Read the model definition and answer for the solid it produces. Units are mm, in the model's axes. Give positions to 0.01 mm unless a question says otherwise; leave off trailing zeros. Write each loop counter-clockwise with the first axis right and the second up, starting at its lowest first coordinate (ties: lowest second). Pieces come first, ordered by that corner, then holes. Notation, with made-up numbers: M 30.5,-3 L 83.5,-3 A21 ccw 83.5,13 Z; hole C 1.25,27 d3. An arc over 180 degrees is marked long. Use a Markdown table: item, result. Add a question column.
Item 1: Given P1, Ø1.5, axis at x = 12, z = 1, coming from the +Y side; P2, Ø1.5, axis at y = 1, z = 1.5, coming from the -X side; P3, Ø1, axis at y = 35.5, z = 1, coming from the -X side, each flat-ended and moving along its own axis, determine where each tip first touches the part or whether it passes through.
Item 2: A cutting plane is placed at A-A on z = 1.7. Determine the outline of the cut face in (x, y).
Item 3: A cutting plane is placed at C-C on y = 25. Determine the outline of the cut face in (x, z).
Item 4: A cutting plane is placed at B-B on x = 6. Determine the outline of the cut face in (y, z), then the cut area to 3 significant figures.
Item 5: Consider probe 1 along X at (y, z) = (48, 0.6); probe 2 along Y at (x, z) = (10, 2.55); probe 3 along Y at (x, z) = (22, 0.5). Determine where each line is inside the solid, lowest interval first. Write a range as [from, to].
Autodesk Inventor part; units mm, degrees
ref_plane "YZ Plane" through (0, 0, 0) normal (1, 0, 0) x (0, 1, 0)
ref_plane "XZ Plane" through (0, 0, 0) normal (0, 1, 0) x (-1, 0, 0)
ref_plane "XY Plane" through (0, 0, 0) normal (0, 0, 1) x (1, 0, 0)
sketch "Sketch1" plane through (0, 0, 0) normal (0, 0, 1) x (1, 0, 0)
  line L0 (0, 0) -> (25, 0)
  line L1 (25, 0) -> (25, 55.5)
  line L2 (25, 55.5) -> (0, 55.5)
  line L3 (0, 55.5) -> (0, 0)
  dimension "d0" = 25
  dimension "d1" = 55.5
extrude "Extrusion1" add sketch "Sketch1" along normal blind 3
sketch "Sketch2" plane through (0, 0, 3) normal (0, 0, 1) x (1, 0, 0)
  line L0 (0, 55.5) -> (0, 0)
  line L1 (25, 55.5) -> (0, 55.5)
  line L2 (0, 0) -> (3, 0)
  line L3 (3, 0) -> (3, 55.5)
  line L4 (3, 55.5) -> (0, 55.5)
  line L5 (0, 55.5) -> (0, 0)
  dimension "d4" = 3
extrude "Extrusion2" cut sketch "Sketch2" against normal through all
sketch "Sketch3" plane through (0, 0, 3) normal (0, 0, 1) x (1, 0, 0)
  point P0 (0, 0)
sketch "Sketch4" plane through (0, 0, 3) normal (0, 0, 1) x (1, 0, 0)
  line L0 (25, 55.5) -> (3, 55.5)
  line L1 (3, 55.5) -> (18.5, 55.5)
  line L2 (18.5, 55.5) -> (18.5, 22.5)
  line L3 (18.5, 22.5) -> (3, 22.5)
  line L4 (3, 22.5) -> (3, 55.5)
  point P0 (0, 0)
  dimension "d7" = 15.5
  dimension "d8" = 33
extrude "Extrusion3" cut sketch "Sketch4" against normal through all
sketch "Sketch5" plane through (0, 0, 3) normal (0, 0, 1) x (1, 0, 0)
  line L0 (3, 0) -> (25, 0)
  line L1 (8, 0) -> (18, 0)
  line L2 (18, 0) -> (18, 3)
  line L3 (18, 3) -> (8, 3)
  line L4 (8, 3) -> (8, 0)
  line L5 (3, 22.5) -> (3, 0)
  line L6 (3, 0) -> (8, 0)
  line L7 (8, 0) -> (8, 3)
  line L8 (8, 3) -> (3, 3)
  line L9 (3, 3) -> (3, 0)
  line L10 (18, 0) -> (25, 0)
  line L11 (25, 0) -> (25, 3)
  line L12 (25, 3) -> (18, 3)
  line L13 (18, 3) -> (18, 0)
  point P0 (0, 0)
  dimension "d11" = 10
  dimension "d12" = 3
  dimension "d13" = 5
extrude "Extrusion4" cut sketch "Sketch5" against normal through all contours L5 L8 L4 L0 | L2 L12 L11 L0
properties part number "hollow_mount"
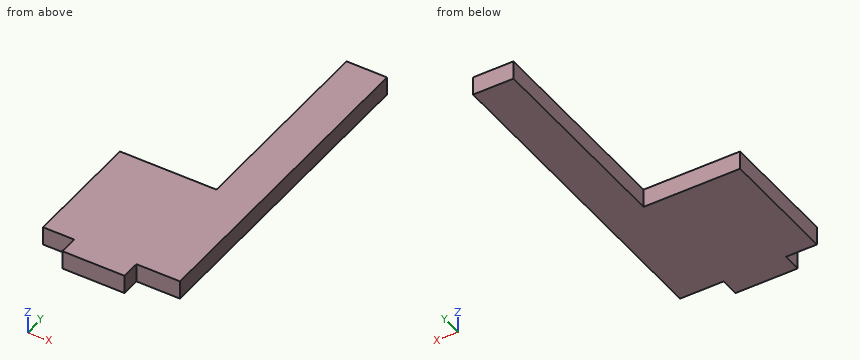
Filled in:
| question | item | result |
|---|---|---|
| 1 | P1 | y = 22.5 |
| 1 | P2 | x = 8 |
| 1 | P3 | x = 18.5 |
| 2 | outline | M 3,3 L 8,3 L 8,0 L 18,0 L 18,3 L 25,3 L 25,55.5 L 18.5,55.5 L 18.5,22.5 L 3,22.5 Z |
| 3 | outline | M 18.5,0 L 25,0 L 25,3 L 18.5,3 Z |
| 4 | outline | M 3,0 L 22.5,0 L 22.5,3 L 3,3 Z |
| 4 | area | 58.5 mm² |
| 5 | probe 1 | [18.5, 25] |
| 5 | probe 2 | [0, 22.5] |
| 5 | probe 3 | [3, 55.5] |
